```python
from build123d import *

# Parameters (mm, degrees)
SKETCH_R             = 2.7
PAD_DEPTH            = 9
SKETCH_MIRRORED_2_R  = 2.7
PAD_MIRRORED_2_DEPTH = 9
POCKET_DEPTH         = 3


with BuildPart() as part:
    # Sketch → Pad (new body)
    with BuildSketch(Plane.XY):
        with BuildLine():
            ThreePointArc((0, -4.2), (2.969848, -2.969848), (4.2, 0))
            Line((4.2, 0), (27, 0))
            Line((27, 0), (27, -14))
            ThreePointArc((21, -20), (25.242641, -18.242641), (27, -14))
            Line((21, -20), (0, -20))
            Line((0, -20), (0, -4.2))
        make_face()
        with Locations((21, -12.5)):
            Circle(SKETCH_R, mode=Mode.SUBTRACT)
    pad = extrude(amount=PAD_DEPTH)

    # Sketch Mirrored 2 → Pad Mirrored 2 (add)
    with BuildSketch(Plane(origin=(0, 0, 0), x_dir=(-1, 0, 0), z_dir=(0, 0, -1))):
        with BuildLine():
            ThreePointArc((0, -4.2), (2.969848, -2.969848), (4.2, 0))
            Line((4.2, 0), (27, 0))
            Line((27, 0), (27, -14))
            ThreePointArc((21, -20), (25.242641, -18.242641), (27, -14))
            Line((21, -20), (0, -20))
            Line((0, -20), (0, -4.2))
        make_face()
        with Locations((21, -12.5)):
            Circle(SKETCH_MIRRORED_2_R, mode=Mode.SUBTRACT)
    pad_mirrored_2 = extrude(amount=-PAD_MIRRORED_2_DEPTH)

    # Mirrored001: Pad, Pad Mirrored 2 across Sketch H_Axis
    add(pad.mirror(Plane.ZX))
    add(pad_mirrored_2.mirror(Plane.ZX))

    # Sketch001 → Pocket (cut)
    with BuildSketch(Plane.XY):
        Polygon((6.5, 3.752777), (0, 7.505553), (-6.5, 3.752777), (-6.5, -3.752777), (0, -7.505553), (6.5, -3.752777), align=None)
    extrude(amount=POCKET_DEPTH, mode=Mode.SUBTRACT)


solid = part.part
```
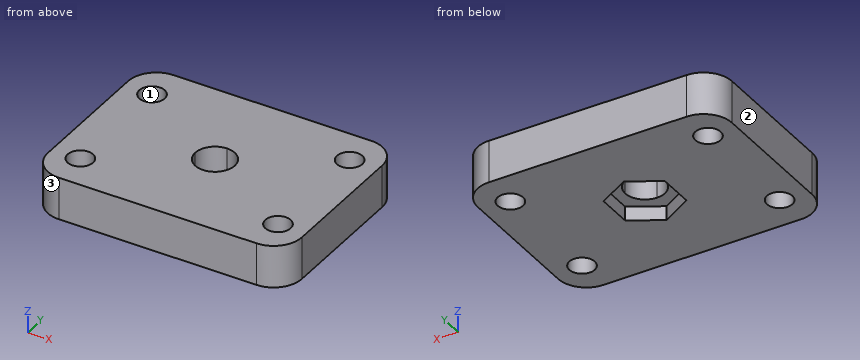
The listing builds one solid part. Answer for the finished solid, in the listing's coordinates (mm). Face numbers are marked on the shaded views. Round coordinates to 2 decimals unless told otherwise and drop trailing zeros. Loops run counter-clockwise (first coordinate to the right, second up) from the corner with the lowest first, then second, coordinate; pieces in that order, holes last. Notation, with made-up numbers: (52.5, 60) - (107.5, 60) arc R30 ccw to (107.5, 90) - close; hole circle Ø11 at (85, 89). An arc over 180 degrees is marked (long way). Return JSON: item names as keys, results as strings. Group by question number.
1. The mould has two halves that part along Y. Classify the marked faces 1, 2 and 3: pulls with the +Y half, pulls with the -Y half, needs draft (parallel to the pull), parting line crosses it, or undercut.
2. The part is cut by section A-A on y = 12.5. Determine the outline of the cut face in (x, z), then the cut area to 3 significant figures.
3. The part is cut by section B-B on z = 6. Determine the outline of the cut face in (x, y).
4. Consider probe 1 along X at (y, z) = (12.5, 8.5); probe 2 along Y at (x, z) = (21, 4.5); probe 3 along X at (y, z) = (14.5, 1). Determine where each line is inside the solid, lowest interval first.
5. Each of these flat-tipped pins is pushed along its axis until it touches: P1, Ø8.5, axis at x = 21, y = 12.5, coming from the -Z side; P2, Ø3, axis at x = -21, y = -12.5, coming from the +Z side. Where does it stop, or does it pass through?
6. The part is cut by section D-D on y = -5. Determine the outline of the cut face in (x, z), then the cut area to 3 significant figures.
7. The part is cut by section C-C on y = -11. Determine the outline of the cut face in (x, z) (3 decimals).
Resolved:
{
 "1": {"face 1": "undercut", "face 2": "needs draft", "face 3": "pulls with the -Y half"},
 "2": {"outline": "(-27, 0) - (-23.7, 0) - (-23.7, 9) - (-27, 9) - close; (-18.3, 0) - (18.3, 0) - (18.3, 9) - (-18.3, 9) - close; (23.7, 0) - (27, 0) - (27, 9) - (23.7, 9) - close", "area": "389 mm²"},
 "3": {"outline": "(-27, -14) arc R6 ccw to (-21, -20) - (21, -20) arc R6 ccw to (27, -14) - (27, 14) arc R6 ccw to (21, 20) - (-21, 20) arc R6 ccw to (-27, 14) - close; hole circle Ø5.4 at (-21, -12.5); hole circle Ø5.4 at (-21, 12.5); hole (-4.2, 0) arc R4.2 ccw to (0, -4.2) arc R4.2 ccw to (4.2, 0) arc R4.2 ccw to (0, 4.2) arc R4.2 ccw to start; hole circle Ø5.4 at (21, -12.5); hole circle Ø5.4 at (21, 12.5)"},
 "4": {"probe 1": "x = -27 to -23.7, -18.3 to 18.3, 23.7 to 27", "probe 2": "y = -20 to -15.2, -9.8 to 9.8, 15.2 to 20", "probe 3": "x = -26.98 to -22.81, -19.19 to 19.19, 22.81 to 26.98"},
 "5": {"P1": "stops at z = 0", "P2": "passes through"},
 "6": {"outline": "(-27, 0) - (-4.34, 0) - (-4.34, 3) - (4.34, 3) - (4.34, 0) - (27, 0) - (27, 9) - (-27, 9) - close", "area": "460 mm²"},
 "7": {"outline": "(-27, 0) - (-23.245, 0) - (-23.245, 9) - (-27, 9) - close; (-18.755, 0) - (18.755, 0) - (18.755, 9) - (-18.755, 9) - close; (23.245, 0) - (27, 0) - (27, 9) - (23.245, 9) - close"}
}
